from build123d import *

# Parameters (mm, degrees)
EXTRUDE_1_DEPTH     = 50
SKETCH_2_R          = 2.5
CUT_EXTRUDE_1_DEPTH = 10
SKETCH_3_R          = 2.5
SKETCH_3_R_2        = 3
CUT_EXTRUDE_2_DEPTH = 10


with BuildPart() as part:
    # Эскиз1 → Бобышка-Вытянуть1 (new body)
    with BuildSketch(Plane(origin=(0, 0, 0), x_dir=(1, 0, 0), z_dir=(0, 1, 0))):
        Polygon((0, 0), (120, 0), (120, 4), (4, 4), (4, 20), (0, 20), (0, 4), align=None)
    extrude(amount=EXTRUDE_1_DEPTH)

    # Эскиз2 → Вырез-Вытянуть1 (cut)
    with BuildSketch(Plane.ZY):
        with Locations((-12, 40)):
            Circle(SKETCH_2_R)
        with Locations((-12, 10)):
            Circle(SKETCH_2_R)
    extrude(amount=-CUT_EXTRUDE_1_DEPTH, mode=Mode.SUBTRACT)

    # Эскиз3 → Вырез-Вытянуть2 (cut)
    with BuildSketch(Plane.XY):
        with Locations((108, 40)):
            Circle(SKETCH_3_R)
        with Locations((108, 10)):
            Circle(SKETCH_3_R)
        with Locations((80, 40)):
            Circle(SKETCH_3_R_2)
    extrude(amount=-CUT_EXTRUDE_2_DEPTH, mode=Mode.SUBTRACT)


solid = part.part
Read the model definition and answer for the solid it produces. Units are mm, in the model's axes. A direction names the side the tool comes from. Give positions to 0.01 mm unless a question says otherwise; leave off trailing zeros. Write each loop counter-clockwise with the first axis right and the second up, starting at its lowest first coordinate (ties: lowest second). Pieces come first, ordered by that corner, then holes. Notation, with made-up numbers: (49, 40.5) - (72, 40.5) arc R32 ccw to (72, 77.5) - close; hole circle Ø11 at (9.25, 82.5). An arc over 180 degrees is marked (long way). Return JSON: item names as keys, results as strings.
Q1. A cutting plane is placed at A-A, the plane z = -12. Determine the outline of the cut face in (x, y), and give its area (3 significant figures).
Reply:
{"outline": "(0, 0) - (4, 0) - (4, 7.5) - (0, 7.5) - close; (0, 12.5) - (4, 12.5) - (4, 37.5) - (0, 37.5) - close; (0, 42.5) - (4, 42.5) - (4, 50) - (0, 50) - close", "area": "160 mm²"}
Q2. Given P1, Ø10, axis at x = 55.5, y = 26.5, coming from the -Z side; P2, Ø3, axis at y = 10, z = -12, coming from the -X side; P3, Ø1.5, axis at y = 40, z = -6, coming from the +X side, each flat-ended and moving along its own axis, determine where each tip first touches the part or whether it passes through.
Reply:
{"P1": "z = -4", "P2": "through", "P3": "x = 4"}
Q3. For a pull along Y with two mould halves and no side action, classify faces 3 (the face through (110.385, 10.751, -1.972)), 4 (the face through (51, 50, -3)), 5 (the face through (51, 0, -3)) as released by +Y, released by -Y, zero draft, split by the parting line, or undercut.
Reply:
{"face 3": "undercut", "face 4": "released by +Y", "face 5": "released by -Y"}
Q4. A cutting plane is placed at B-B, the plane y = 10. Determine the outline of the cut face in (x, z).
Reply:
{"outline": "(0, -20) - (4, -20) - (4, -14.5) - (0, -14.5) - close; (0, -9.5) - (4, -9.5) - (4, -4) - (105.5, -4) - (105.5, 0) - (0, 0) - close; (110.5, -4) - (120, -4) - (120, 0) - (110.5, 0) - close"}
Q5. A cutting plane is placed at C-C, the plane y = 40. Determine the outline of the cut face in (x, z).
Reply:
{"outline": "(0, -20) - (4, -20) - (4, -14.5) - (0, -14.5) - close; (0, -9.5) - (4, -9.5) - (4, -4) - (77, -4) - (77, 0) - (0, 0) - close; (83, -4) - (105.5, -4) - (105.5, 0) - (83, 0) - close; (110.5, -4) - (120, -4) - (120, 0) - (110.5, 0) - close"}
Q6. For faces 1 (the face through (110.385, 40.751, -1.972)), 2 (the face through (63, 25, -4)), determine the directions among +Z, -Z, +X, -X, +Y, -Y from which every point of the face is accessible in a straight line to the end or side of a thin tool.
Reply:
{"face 1": "+Z, -Z", "face 2": "-Z, +X, +Y, -Y"}
Q7. Consider line 1 along Y through (x, z) = (108, -2.15); line 2 along Z through (x, y) = (98.5, 6.5); line 3 along X through (y, z) = (18, -12.5). Determine where each line is inside the solid, lowest interval first. Write a range as [from, to].
Reply:
{"line 1": "[0, 7.5], [12.5, 37.5], [42.5, 50]", "line 2": "[-4, 0]", "line 3": "[0, 4]"}
Q8. A cutting plane is placed at D-D, the plane x = 108. Determine the outline of the cut face in (y, z).
Reply:
{"outline": "(0, -4) - (7.5, -4) - (7.5, 0) - (0, 0) - close; (12.5, -4) - (37.5, -4) - (37.5, 0) - (12.5, 0) - close; (42.5, -4) - (50, -4) - (50, 0) - (42.5, 0) - close"}
